Autodesk Inventor part; units mm, degrees
ref_plane "YZ Plane" through (0, 0, 0) normal (1, 0, 0) x (0, 1, 0)
ref_plane "XZ Plane" through (0, 0, 0) normal (0, 1, 0) x (-1, 0, 0)
ref_plane "XY Plane" through (0, 0, 0) normal (0, 0, 1) x (1, 0, 0)
sketch "Sketch1" plane through (0, 0, 0) normal (1, 0, 0) x (0, 1, 0)
  line L0 (48, 50) -> (-48, 50)
  line L1 (-48, 50) -> (-48, -50)
  line L2 (-48, -50) -> (48, -50)
  line L3 (48, -50) -> (48, 50)
  point P0 (0, 0)
  dimension "d0" = 96
  dimension "d1" = 100
  dimension "d2" = 50
  dimension "d3" = 48
extrude "Extrusion1" add sketch "Sketch1" along normal blind 1.5
sketch "Sketch2" plane through (0, -48, 50) normal (0, 0, 1) x (1, 0, 0)
  line L0 (0, 96) -> (1.5, 96)
  line L1 (1.5, 96) -> (-7, 96)
  line L2 (-7, 96) -> (-7, 0)
  line L3 (-7, 0) -> (1.5, 0)
  line L4 (1.5, 0) -> (1.5, 96)
  point P0 (0, 48)
  dimension "d6" = 8.5
  dimension "d7" = 96
extrude "Extrusion2" add sketch "Sketch2" against normal blind 1.5
mirror "Mirror1" about plane through (0, 0, 0) normal (0, 0, 1) of "Extrusion2"
fillet "Fillet1" radius 0.5 2 edges at (1.5, 0, 50) (1.5, 0, -50)
sketch "Sketch9" plane through (-7, -48, 48.5) normal (0, -1, 0) x (1, 0, 0)
  arc A0 (8, -98.5) -> (8.5, -98) centre (8, -98) ccw
  line L0 (8.5, 1) -> (8.5, -98)
  arc A1 (8.5, 1) -> (8, 1.5) centre (8, 1) ccw
  line L1 (0, 1.5) -> (8, 1.5)
  line L2 (0, 1.5) -> (0, 0)
  line L3 (7, 0) -> (0, 0)
  line L4 (7, 0) -> (7, -97)
  line L5 (7, -97) -> (0, -97)
  line L6 (0, -98.5) -> (0, -97)
  line L7 (0, -98.5) -> (8, -98.5)
  point P0 (7, -48.5)
extrude "Extrusion6" add sketch "Sketch9" along normal blind 56.75
sketch "Sketch10" plane through (-7, 48, 48.5) normal (0, 1, 0) x (1, 0, 0)
  arc A0 (8.5, 98) -> (8, 98.5) centre (8, 98) ccw
  line L0 (0, 98.5) -> (8, 98.5)
  line L1 (0, 98.5) -> (0, 97)
  line L2 (0, 97) -> (7, 97)
  line L3 (7, 97) -> (7, 0)
  line L4 (0, 0) -> (7, 0)
  line L5 (0, -1.5) -> (0, 0)
  line L6 (8, -1.5) -> (0, -1.5)
  arc A1 (8, -1.5) -> (8.5, -1) centre (8, -1) ccw
  line L7 (8.5, 98) -> (8.5, -1)
  point P0 (7, 48.5)
extrude "Extrusion7" add sketch "Sketch10" along normal blind 56.75
sketch "Sketch11" plane through (1.5, 0, 0) normal (1, 0, 0) x (0, 0, -1)
  circle A0 centre (35, -100.75) radius 3
  circle A1 centre (-35, -100.75) radius 3
  circle A2 centre (-30, -48) radius 3
  circle A3 centre (30, -48) radius 3
  circle A4 centre (30, 48) radius 3
  circle A5 centre (-30, 48) radius 3
  circle A6 centre (35, 100.75) radius 3
  circle A7 centre (-35, 100.75) radius 3
  point P0 (0, 0)
hole "Hole5" at (1.5, -100.75, -35) at (1.5, -100.75, 35) at (1.5, -48, 30) at (1.5, -48, -30) at (1.5, 48, 30) at (1.5, 48, -30) at (1.5, 100.75, 35) at (1.5, 100.75, -35) direction (-1, 0, 0) diameter 3.454 end through all
properties part number "memesat shear panel type 1" material "Aluminum 6061"
CAD build for the part. Positions are in the model's coordinates, mm. A direction names the side the tool comes from. Give positions to 0.01 mm unless a question says otherwise; leave off trailing zeros. Write each loop counter-clockwise with the first axis right and the second up, starting at its lowest first coordinate (ties: lowest second). Pieces come first, ordered by that corner, then holes. Notation, with made-up numbers: M 81,6.5 L 121,6.5 A19 cw 121,18.5 Z; hole C 35.5,69 d4. An arc over 180 degrees is marked long. Put each result on its own line as item: value. Start each with the question number.
(1) Band-saw the part on B-B, the plane y = 88. Write the cut outline in (x, z), and give its area (3 significant figures).
(2) Flat gauge pins, fed straight in: pin 1 Ø10 at (y, z) = (64, 31) entering from -X; pin 2 Ø3 at (y, z) = (-48, 30) entering from -X (1 decimal); pin 3 Ø5.5 at (y, z) = (100.75, 35) entering from +X. Where does each tip first touch, or does it go through?
(3) Mould opens along Z. For faces 3 (the face through (1.5, -1, -1)), 4 (the face through (0, -1, -1)), 5 (the face through (-3, -1, -50)), 6 (the face through (-4, -1, -48.5)) say: +Z half, -Z half, draft (parallel to the pull), parting line (faces both ways), or undercut.
(4) Which spindle directions (+Z, -Z, +X, -X, +Y, -Y) get a long thin tool onto all of the face, cutting with end or side? Do faces 1 (the face through (-3, -1, 50)), 2 (the face through (-4, -1, 48.5)). Say none if no direction does.
(5) Band-saw the part on C-C, the plane z = -12. Write the cut outline in (x, y).
(6) Probe L1, parallel to Y at x = 1.05, z = 30; L2, parallel to Z at x = 0.75, y = 100.75; L3, parallel to Z at x = 0.55, y = 48. List the from-to ranges inside material, lowest first.
(7) Band-saw the part on A-A, the plane x = -5.5. Write the cut outline in (y, z), and give its area (4 significant figures).
Response values:
1. outline: M -7,-50 L 1,-50 A0.5 ccw 1.5,-49.5 L 1.5,49.5 A0.5 ccw 1,50 L -7,50 L -7,48.5 L 0,48.5 L 0,-48.5 L -7,-48.5 Z
1. area: 171 mm2
2. pin 1: stops at x = 0
2. pin 2: passes through
2. pin 3: stops at x = 1.5
3. face 3: draft
3. face 4: undercut
3. face 5: -Z half
3. face 6: undercut
4. face 1: +Z, +X, -X, +Y, -Y
4. face 2: -X, +Y, -Y
5. outline: M 0,-104.75 L 1.5,-104.75 L 1.5,104.75 L 0,104.75 Z
6. L1: y = -104.75 to -49.73, -46.27 to 46.27, 49.73 to 104.75
6. L2: z = -50 to -36.73, -33.27 to 33.27, 36.73 to 50
6. L3: z = -50 to -31.73, -28.27 to 28.27, 31.73 to 50
7. outline: M -104.75,-50 L 104.75,-50 L 104.75,-48.5 L -104.75,-48.5 Z; M -104.75,48.5 L 104.75,48.5 L 104.75,50 L -104.75,50 Z
7. area: 628.5 mm2
